Input: part model. Units: mm. Frame: model coordinates. Round coordinates to 2 decimals unless told otherwise and drop trailing zeros.
(1) First-contact query: pin 1 Ø10 at (x, y) = (105, -57) entering from -Z; pin 2 Ø14.5 at (x, y) = (325, -325) entering from -Z; pin 3 Ø11.5 at (x, y) = (50, -50) entering from +Z; pin 4 Ø5.5 at (x, y) = (325, -125) entering from +Z. Flat tips, straight axial feed; report the tip coordinate or a pass-through.
(2) Line query: line 1 (Y direction, x = 325, z = 5.95); line 2 (X direction, y = -50, z = 1.7); line 3 (Y direction, x = 400, z = 2.25). Output: solid intervals per line, ascending.
(3) Draft query along Y for faces 1 (the face through (53.743, -52.87, 3.757)), 2 (the face through (222, -222, 8)). Return one class per face: released by +Y, released by -Y, zero draft, split by the parting line, or undercut.
from build123d import *

# Parameters (mm, degrees)
F0_W           = 450
F0_H           = 450
F1_DEPTH       = 8
F3_D           = 9
F3_CSINK_D     = 17.92
F3_CSINK_ANGLE = 90
F5_D           = 9
F5_CSINK_D     = 17.92
F5_CSINK_ANGLE = 90


with BuildPart() as f1:
    # F0 (on Top) → F1 (new body)
    with BuildSketch(Plane.XY):
        with Locations((225, -225)):
            Rectangle(F0_W, F0_H)
    extrude(amount=F1_DEPTH)

    # F3 (through all)
    with Locations(Plane.XY.offset(8)):
        with Locations((50, -400), (400, -400), (400, -50), (50, -50)):
            CounterSinkHole(F3_D / 2, F3_CSINK_D / 2, counter_sink_angle=F3_CSINK_ANGLE)

    # F5 (through all)
    with Locations(Plane(origin=(0, 0, 0), x_dir=(1, 0, 0), z_dir=(0, 0, -1))):
        with Locations((125, 325), (325, 125), (325, 325), (125, 125)):
            CounterSinkHole(F5_D / 2, F5_CSINK_D / 2, counter_sink_angle=F5_CSINK_ANGLE)


solid = f1.part
Reported:
1. pin 1: stops at z = 0
1. pin 2: stops at z = 1.71
1. pin 3: stops at z = 4.79
1. pin 4: passes through
2. line 1: y = -450 to -329.5, -320.5 to -129.5, -120.5 to 0
2. line 2: x = 0 to 45.5, 54.5 to 395.5, 404.5 to 450
2. line 3: y = -450 to -404.5, -395.5 to -54.5, -45.5 to 0
3. face 1: undercut
3. face 2: zero draft
